```python
from build123d import *

# Parameters (mm, degrees)
F1_DEPTH = 62.23
F3_DEPTH = 62.23
F4_DEPTH = 10.795
F5_DEPTH = 10.795


with BuildPart() as f1:
    # F0 (on Top) → F1 (new body)
    with BuildSketch(Plane.XY):
        Polygon((-7.3319007784, -0.081020421), (-3.5957846464, -6.3901225426), (3.736116132, -6.3091021217), (7.3319007784, 0.081020421), (3.5957846464, 6.3901225426), (-3.736116132, 6.3091021217), align=None)
    extrude(amount=F1_DEPTH)

    # F2 (on face) → F3 (cut, through all)
    with BuildSketch(Plane(origin=(0, 0, 0), x_dir=(1, 0, 0), z_dir=(0, 0, -1))):
        with BuildLine():
            ThreePointArc((-6.2100646879, 1.9754418492), (-4.6811988128, 2.6884458628), (-4.7909795689, 4.3718215705))
            Line((-4.7909795689, 4.3718215705), (-6.2100646879, 1.9754418492))
        make_face()
        with BuildLine():
            Line((1.3906187564, 6.3350208009), (-1.3942495189, 6.3657947035))
            ThreePointArc((-1.3942495189, 6.3657947035), (-0.0123369925, 5.3982600234), (1.3906187564, 6.3350208009))
        make_face()
        with BuildLine():
            Line((6.1815983253, 1.9631992305), (4.815815169, 4.3903528543))
            ThreePointArc((4.815815169, 4.3903528543), (4.6688618202, 2.7098141606), (6.1815983253, 1.9631992305))
        make_face()
        with BuildLine():
            Line((4.7909795689, -4.3718215705), (6.2100646879, -1.9754418492))
            ThreePointArc((6.2100646879, -1.9754418492), (4.6811988128, -2.6884458628), (4.7909795689, -4.3718215705))
        make_face()
        with BuildLine():
            ThreePointArc((1.3942495189, -6.3657947035), (0.0123369925, -5.3982600234), (-1.3906187564, -6.3350208009))
            Line((-1.3906187564, -6.3350208009), (1.3942495189, -6.3657947035))
        make_face()
        with BuildLine():
            ThreePointArc((-4.815815169, -4.3903528543), (-4.6688618202, -2.7098141606), (-6.1815983253, -1.9631992305))
            Line((-6.1815983253, -1.9631992305), (-4.815815169, -4.3903528543))
        make_face()
    extrude(amount=-F3_DEPTH, mode=Mode.SUBTRACT)

    # F4 (add): a face of the model
    f4_faces = [f1.faces().sort_by_distance(p)[0] for p in [
        (0, 0, 62.23),
    ]]
    extrude(f4_faces, amount=F4_DEPTH)

    # F5 (cut): a face of the model
    f5_faces = [f1.faces().sort_by_distance(p)[0] for p in [
        (0, 0, 73.025),
    ]]
    extrude(f5_faces, amount=-F5_DEPTH, mode=Mode.SUBTRACT)


solid = f1.part
```
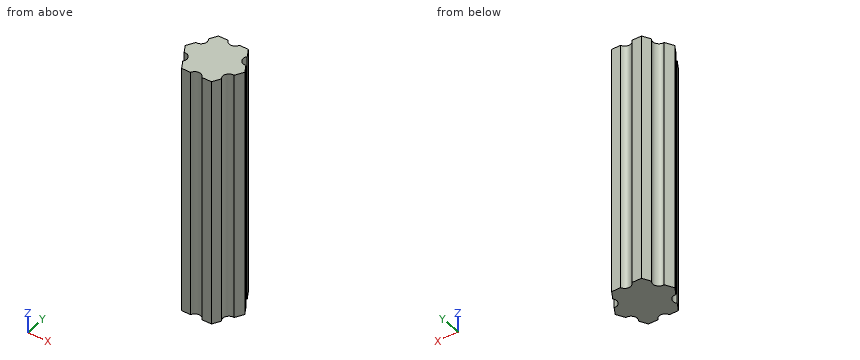
For this review, take the finished solid that the model builds, in its own axes (mm). Give positions to 0.01 mm unless a question says otherwise; leave off trailing zeros. Write each loop counter-clockwise with the first axis right and the second up, starting at its lowest first coordinate (ties: lowest second). Pieces come first, ordered by that corner, then holes.
Item 1: Take a section at C-C (y = 3.5). Give the boundary of the cut face in (x, z).
Item 2: Take a section at A-A (z = 52). Give the boundary of the cut face in (x, y).
Item 3: Wall thickness on probe 1 along Y at (x, z) = (2.75, 6); probe 2 along Y at (x, z) = (-2, 8); probe 3 along X at (y, z) = (2.5, 49): over which ranges is each line inside the solid? List them lowest first.
Item 4: Take a section at B-B (x = 5.5). Give the boundary of the cut face in (y, z).
Item 5: Insertion check: P1, Ø6, axis at x = -0.5, z = 53, coming from the +Y side. The pin has a flat end and moves straight along its axis. Give the tip position at first contact, or say it passes through.
Established:
1. outline: (-4.48, 0) - (4.47, 0) - (4.47, 62.23) - (-4.48, 62.23) - close
2. outline: (-7.33, -0.08) - (-6.21, -1.98) arc R1.49 cw to (-4.79, -4.37) - (-3.6, -6.39) - (-1.39, -6.37) arc R1.49 cw to (1.39, -6.34) - (3.74, -6.31) - (4.82, -4.39) arc R1.49 cw to (6.18, -1.96) - (7.33, 0.08) - (6.21, 1.98) arc R1.49 cw to (4.79, 4.37) - (3.6, 6.39) - (1.39, 6.37) arc R1.49 cw to (-1.39, 6.34) - (-3.74, 6.31) - (-4.82, 4.39) arc R1.49 cw to (-6.18, 1.96) - close
3. probe 1: y = -6.32 to 6.38
3. probe 2: y = -6.37 to 6.33
3. probe 3: x = -4.81 to 4.81
4. outline: (-2.02, 0) - (2.03, 0) - (2.03, 62.23) - (-2.02, 62.23) - close
5. P1: stops at y = 6.38
